Geometry: final body of the model. Coordinates: model frame, mm. A direction names the side the tool comes from. Give positions to 0.01 mm unless a question says otherwise; leave off trailing zeros. Write each loop counter-clockwise with the first axis right and the second up, starting at its lowest first coordinate (ties: lowest second). Pieces come first, ordered by that corner, then holes. Notation, with made-up numbers: (87.25, 70.25) -> (111.25, 70.25) arc R32 ccw to (111.25, 106.25) -> close; hole circle Ø11 at (61, -19). An arc over 180 degrees is marked (long way). Answer as a JSON object with one key per item and string values. Group by question number.
(1) Section query D-D on x = -0.4. Output: boundary loops of the cut face in (y, z) (3 decimals), plus the area to 3 significant figures.
(2) Set-up query: faces 1 (the face through (0.507, 0.976, -0.217)), 2 (the face through (3, -2, 0)). Return all of +Z, -Z, +X, -X, +Y, -Y with unobstructed straight access to the full face (end or side cutting, diameter ignored); none if empty.
(3) Section query C-C on z = -4.5. Output: boundary loops of the cut face in (x, y).
(4) Contact query for flat-ended pins moving along their axis: pin 1 Ø2 at (x, z) = (2, 3) entering from -Y; pin 2 Ø1 at (x, y) = (1, 2) entering from +Z; pin 3 Ø2.5 at (y, z) = (0, 0) entering from +X; pin 4 Ø1.5 at (x, z) = (2, -1) entering from +Y. Output: stop coordinate, or through.
(5) Section query A-A on z = 0. Output: boundary loops of the cut face in (x, y) (3 decimals).
(6) Material intervals for probe 1 along Y at (x, z) = (2.9, 0); probe 2 along Y at (x, z) = (2.3, -4.5); probe 3 along Z at (x, y) = (2.55, -5.5), sorted ascending.
from build123d import *

# Parameters (mm, degrees)
BASPROSKE_W         = 4
BASPROSKE_H         = 7.875
TOOTHCUT_DEPTH      = 12.833480046
TEETHCUTS_COUNT     = 12
TEETHCUTS_ANGLE     = 330
BORSKE_R            = 1
BORE_DEPTH          = 50.0000508
SKETCH1_R           = 3.375
SKETCH1_R_2         = 2.375
BOSS_EXTRUDE1_DEPTH = 2
SKETCH2_R           = 2
CUT_EXTRUDE1_DEPTH  = 3


with BuildPart() as part:
    # BasProSke → Base-Revolve (revolve)
    with BuildSketch(Plane(origin=(0, 0, 0), x_dir=(1, 0, 0), z_dir=(0, 1, 0)), mode=Mode.PRIVATE) as base_revolve_sk:
        with Locations((2, 3.9375)):
            Rectangle(BASPROSKE_W, BASPROSKE_H)
    revolve(base_revolve_sk.sketch.rotate(Axis((-10, 0, 0), (1, 0, 0)), 180), axis=Axis((-10, 0, 0), (1, 0, 0)))

    # TooCutSke → ToothCut (cut, through all)
    with BuildSketch(Plane(origin=(0, 0, 0), x_dir=(0, 0, -1), z_dir=(1, 0, 0))):
        with BuildLine():
            ThreePointArc((0.631439839, 5.305305014), (0, 5.34275), (-0.631439839, 5.305305014))
            ThreePointArc((-0.631439839, 5.305305014), (-0.93992237, 6.654932089), (-1.876748184, 7.674251521))
            ThreePointArc((-1.876748184, 7.674251521), (0, 7.9004), (1.876748184, 7.674251521))
            ThreePointArc((1.876748184, 7.674251521), (0.93992237, 6.654932089), (0.631439839, 5.305305014))
        make_face()
    toothcut = extrude(amount=TOOTHCUT_DEPTH, mode=Mode.SUBTRACT)

    # TeethCuts: ToothCut ×12 about axis
    teethcuts_axis = Axis((-10, 0, 0), (1, 0, 0))
    for i in range(1, TEETHCUTS_COUNT):
        add(toothcut.rotate(teethcuts_axis, i * TEETHCUTS_ANGLE / (TEETHCUTS_COUNT - 1)), mode=Mode.SUBTRACT)

    # BorSke → Bore (cut, symmetric)
    with BuildSketch(Plane(origin=(0, 0, 0), x_dir=(0, 0, -1), z_dir=(1, 0, 0))):
        with Locations(Location((0, 0, 0), (0, 0, 180))):
            Circle(BORSKE_R)
    extrude(amount=BORE_DEPTH, both=True, mode=Mode.SUBTRACT)

    # Sketch1 → Boss-Extrude1 (add)
    with BuildSketch(Plane.ZY):
        with Locations(Location((0, 0, 0), (0, 0, 180))):
            Circle(SKETCH1_R)
        Circle(SKETCH1_R_2, mode=Mode.SUBTRACT)
    extrude(amount=BOSS_EXTRUDE1_DEPTH)

    # Sketch2 → Cut-Extrude1 (cut)
    with BuildSketch(Plane(origin=(4, 0, 0), x_dir=(0, 0, -1), z_dir=(1, 0, 0))):
        Circle(SKETCH2_R)
    extrude(amount=-CUT_EXTRUDE1_DEPTH, mode=Mode.SUBTRACT)


solid = part.part
Answer list:
{
 "1": {"outline": "circle Ø6.75 at (0, 0); hole circle Ø4.75 at (0, 0)", "area": "18.1 mm2"},
 "2": {"face 1": "+X, -X", "face 2": "+X"},
 "3": {"outline": "(0, -5.48) -> (4, -5.48) -> (4, -3.33) -> (0, -3.33) -> close; (0, -2.88) -> (4, -2.88) -> (4, 2.88) -> (0, 2.88) -> close; (0, 3.33) -> (4, 3.33) -> (4, 5.48) -> (0, 5.48) -> close"},
 "4": {"pin 1": "y = -7.62", "pin 2": "z = 7.66", "pin 3": "x = 1", "pin 4": "y = 7.59"},
 "5": {"outline": "(-2, -3.375) -> (0, -3.375) -> (0, -5.343) -> (4, -5.343) -> (4, -2) -> (1, -2) -> (1, -1) -> (0, -1) -> (0, -2.375) -> (-2, -2.375) -> close; (-2, 2.375) -> (0, 2.375) -> (0, 1) -> (1, 1) -> (1, 2) -> (4, 2) -> (4, 5.343) -> (0, 5.343) -> (0, 3.375) -> (-2, 3.375) -> close"},
 "6": {"probe 1": "-5.34 to -2, 2 to 5.34", "probe 2": "-5.48 to -3.33, -2.88 to 2.88, 3.33 to 5.48", "probe 3": "-5.64 to -4.54, -2.38 to -0.63, 0.63 to 2.38, 4.54 to 5.64"}
}
